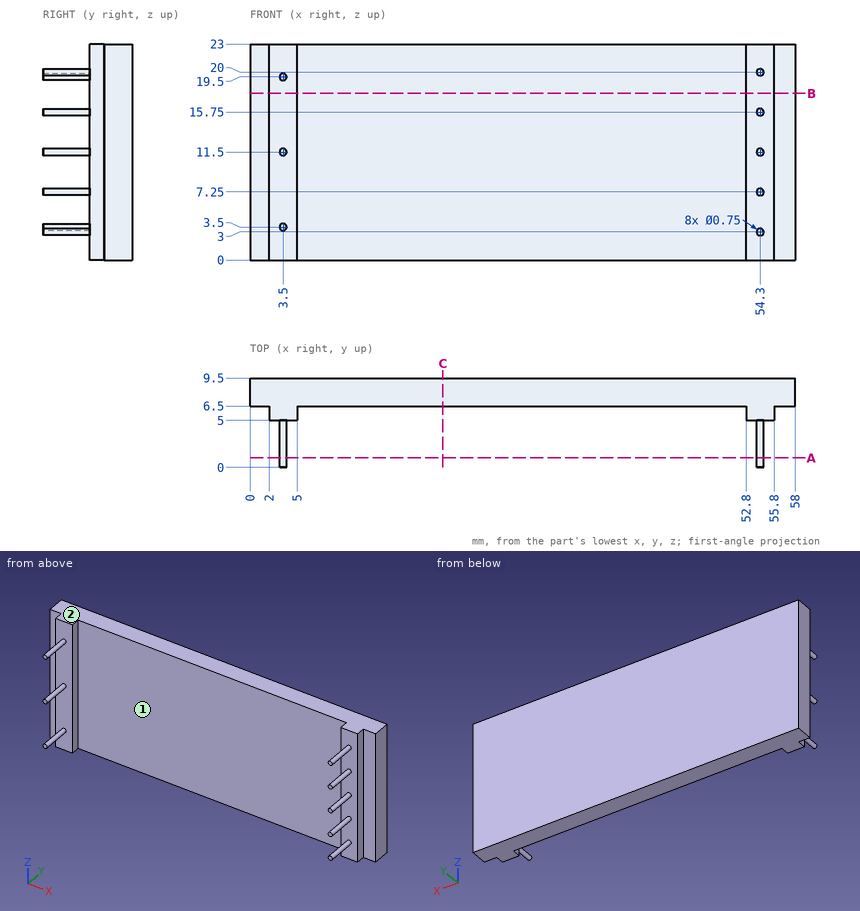
Job drawing, mm, ordinate dimensions from the low corner. One solid piece. Coordinates: 2 decimals unless noted, no trailing zeros. Order: outer loops, then holes, each group sorted by start corner. A loop starts at its lowest first (then second) coordinate and runs counter-clockwise, first axis right, second up. Notation, with made-up numbers: (47, 60) - (58, 60) arc R6 ccw to (58, 71) - close; hole circle Ø9 at (47.5, 65). An arc over 180 degrees is marked (long way). Use CSV: the item, a comma, the result in double quotes.
Item 1: Saw through at A-A on y = 1. Give the cut face in (x, z) (3 decimals), and give its area (3 significant figures).
Solved:
outline,"circle Ø0.75 at (3.5, 3.5); circle Ø0.75 at (3.5, 11.5); circle Ø0.75 at (3.5, 19.5); circle Ø0.75 at (54.3, 3); circle Ø0.75 at (54.3, 7.25); circle Ø0.75 at (54.3, 11.5); circle Ø0.75 at (54.3, 15.75); circle Ø0.75 at (54.3, 20)"
area,"3.53 mm²"
Item 2: Saw through at B-B on z = 17.75. Give the cut face in (x, y).
Solved:
outline,"(0, 6.5) - (2, 6.5) - (2, 5) - (5, 5) - (5, 6.5) - (52.8, 6.5) - (52.8, 5) - (55.8, 5) - (55.8, 6.5) - (58, 6.5) - (58, 9.5) - (0, 9.5) - close"
Item 3: Drop flat-ended pins along their axis: P1, Ø1.8, axis at x = 57, z = 14, coming from the -Y side; P2, Ø3.5, axis at x = 3.5, z = 15.5, coming from the -Y side; P3, Ø0.8, axis at y = 6, z = 8.5, coming from the +X side; P4, Ø1.6, axis at y = 6, z = 11.5, coming from the -X side. Give the stop position or say it passes through.
Solved:
P1,"stops at y = 6.5"
P2,"stops at y = 5"
P3,"stops at x = 55.8"
P4,"stops at x = 0"
Item 4: Probe probe 1 along X at (y, z) = (5.5, 22.25); probe 2 along Y at (x, z) = (36.5, 18.5); probe 3 along X at (y, z) = (0.5, 15.75) (3 decimals). List the from-to ranges inside material, lowest first.
Solved:
probe 1,"x = 2 to 5, 52.8 to 55.8"
probe 2,"y = 6.5 to 9.5"
probe 3,"x = 53.925 to 54.675"
Item 5: Saw through at C-C on x = 20.5. Give the cut face in (y, z).
Solved:
outline,"(6.5, 0) - (9.5, 0) - (9.5, 23) - (6.5, 23) - close"
Item 6: Mould opens along X. For the marked faces 1 and 2 say: +X half, -X half, draft (parallel to the pull), parting line (faces both ways), or undercut.
Solved:
face 1,"undercut"
face 2,"draft"
